Could you check a few things on this model? Use its own coordinates, in mm. A direction names the side the tool comes from. Give positions to 0.01 mm unless a question says otherwise; leave off trailing zeros. Order: outer loops, then holes, each group sorted by start corner. A loop starts at its lowest first (then second) coordinate and runs counter-clockwise, first axis right, second up. Notation, with made-up numbers: M -20.75,54.25 L 17.25,54.25 A9 ccw 17.25,62.25 Z; hole C 67.25,-10.5 d8. An arc over 180 degrees is marked long. Use a Markdown table: item, result. Add a question column.
Item 1: If we mould it in two halves opening along X, with no side actions, what happens to faces 6 (the face through (-6, 6, -22)), 7 (the face through (18.5, 18, 27)), 8 (the face through (11.491, 8, 23))? For each: released by +X, released by -X, zero draft, split by the parting line, or undercut.
Item 2: If I drill on L1, parallel to X at y = 1.25, z = -11; L2, parallel to Z at x = -12, y = 3.25; L3, parallel to X at y = 3, z = 23, over which ranges is the centre line in solid material (lowest first)? Write a range as from..to.
Item 3: Suppose I cut it at B-B on y = 10.25. Write out the boundary of the cut face in (x, z).
Item 4: For faces 1 (the face through (1, 2, 20.9)), 2 (the face through (-6, 11.5, 27)), 3 (the face through (-24, 2, -2)), 4 (the face through (11.5, 2, -2)), 5 (the face through (-7, 16, 24.5)), which set-ups out of +Z, -Z, +X, -X, +Y, -Y let a thin tool reach every point of the face, with its end or its side?
Item 5: Suppose I cut it at D-D on x = -6.5. Write out the boundary of the cut face in (y, z).
Item 6: Suppose I cut it at A-A on y = 6.5. Count the separate pieces of the cut face and the enclosed holes in it, plus the area to 3 significant figures.
Item 7: Suppose I cut it at C-C on z = -13. Write out the boundary of the cut face in (x, y), plus the area to 3 significant figures.
Item 8: I'm going to push flat-ended pins straight in: pin 1 Ø5 at (x, z) = (-36.5, 26) entering from +Y; pin 2 Ø10 at (x, z) = (-2.5, 5) entering from -Y; pin 3 Ø2 at (x, y) = (-4.5, 5) entering from +Z; pin 4 Ø8 at (x, z) = (17, 1.5) entering from +Y. Where does each tip first touch, or does it pass through?
from build123d import *

# Parameters (mm, degrees)
ESQUISSE1_W             = 35.5
ESQUISSE1_H             = 56
ESQUISSE1_W_2           = 20.1
ESQUISSE1_H_2           = 40.9
BOSS_EXTRU_1_DEPTH      = 4
BOSS_EXTRU_2_DEPTH      = 4
BOSS_EXTRU_5_DEPTH      = 4
ESQUISSE10_W            = 17
ESQUISSE10_H            = 13
BOSS_EXTRU_6_DEPTH      = 7
ESQUISSE11_R            = 3
ENL_V_MAT_EXTRU_1_DEPTH = 7
CONG_1_R                = 0.5
ESQUISSE12_W            = 8
ESQUISSE12_H            = 10.6
ENL_V_MAT_EXTRU_2_DEPTH = 11.5


with BuildPart() as part:
    # Esquisse1 → Boss.-Extru.1 (new body)
    with BuildSketch(Plane(origin=(0, 0, 0), x_dir=(1, 0, 0), z_dir=(0, 1, 0))):
        with Locations((-6.25, -0.5)):
            Rectangle(ESQUISSE1_W, ESQUISSE1_H)
        with Locations((-6.05, -0.45)):
            Rectangle(ESQUISSE1_W_2, ESQUISSE1_H_2, mode=Mode.SUBTRACT)
    extrude(amount=BOSS_EXTRU_1_DEPTH)

    # Esquisse5 → Boss.-Extru.2 (add)
    with BuildSketch(Plane.XY.offset(28.5)):
        Polygon((-6.25, 8), (-6.25, 4), (-6.25, 0), (11.5, 0), (11.5, 13), (18.5, 13), (18.5, 18), (18.5, 23), (-6.25, 23), (-6.25, 18), align=None)
    boss_extru_2 = extrude(amount=-BOSS_EXTRU_2_DEPTH)

    # Symétrie1: Boss.-Extru.2 across plane
    add(boss_extru_2.mirror(Plane(origin=(-6.25, 4, 24.5), x_dir=(0, 0, 1), z_dir=(-1, 0, 0))))

    # Esquisse9 → Boss.-Extru.5 (add)
    with BuildSketch(Plane(origin=(0, 4, 0), x_dir=(-1, 0, 0), z_dir=(0, -1, 0))):
        Polygon((18.5, -25.5), (18.5, -23), (18.5, 20), (18.5, 22), (-6, 22), (-6, -25.5), align=None)
    extrude(amount=-BOSS_EXTRU_5_DEPTH)

    # Esquisse10 → Boss.-Extru.6 (add)
    with BuildSketch(Plane.XY.offset(28.5)):
        with Locations((19.990927164, 6.5)):
            Rectangle(ESQUISSE10_W, ESQUISSE10_H)
    boss_extru_6 = extrude(amount=-BOSS_EXTRU_6_DEPTH)

    # Symétrie2: Boss.-Extru.6 across plane
    add(boss_extru_6.mirror(Plane(origin=(-6.25, 0, 0), x_dir=(0, 0, 1), z_dir=(1, 0, 0))))

    # Esquisse11 → Enlèv. mat.-Extru.1 (cut)
    with BuildSketch(Plane(origin=(0, 0, 21.5), x_dir=(-1, 0, 0), z_dir=(0, 0, -1))):
        with Locations((-19.990927164, 6.5)):
            Circle(ESQUISSE11_R)
    enl_v_mat_extru_1 = extrude(amount=-ENL_V_MAT_EXTRU_1_DEPTH, mode=Mode.SUBTRACT)

    # Symétrie3: Enlèv. mat.-Extru.1 across plane
    add(enl_v_mat_extru_1.mirror(Plane(origin=(-6.25, 0, 0), x_dir=(0, 0, 1), z_dir=(1, 0, 0))), mode=Mode.SUBTRACT)

    # Congé1
    cong_1_edges = [part.edges().sort_by_distance(p)[0] for p in [
        (19.995463582, 0, 21.5),
        (11.490927164, 8.5, 24.5),
        (19.990927164, 13, 21.5),
        (28.490927164, 6.5, 21.5),
        (-21.245463582, 4, 24.5),
        (-23.990927164, 8.5, 24.5),
        (-32.495463582, 0, 21.5),
        (-40.990927164, 6.5, 21.5),
        (-32.490927164, 13, 21.5),
        (14.995463582, 13, 24.5),
        (18.5, 13, 26.5),
        (-6.25, 23, 24.5),
        (18.5, 18, 24.5),
        (-31, 13, 26.5),
        (-27.495463582, 13, 24.5),
        (-31, 18, 24.5),
        (8.745463582, 4, 24.5),
        (-6.25, 8, 24.5),
        (6, 6, 24.5),
        (-18.5, 6, 24.5),
    ]]
    fillet(cong_1_edges, radius=CONG_1_R)

    # Esquisse12 → Enlèv. mat.-Extru.2 (cut)
    with BuildSketch(Plane.XZ):
        with Locations((-6.05, 23.2)):
            Rectangle(ESQUISSE12_W, ESQUISSE12_H)
    extrude(amount=-ENL_V_MAT_EXTRU_2_DEPTH, mode=Mode.SUBTRACT)


solid = part.part
Findings below:
| question | item | result |
|---|---|---|
| 1 | face 6 | zero draft |
| 1 | face 7 | released by +X |
| 1 | face 8 | undercut |
| 2 | L1 | x = -24..-16.1, 4..11.5 |
| 2 | L2 | z = -27.5..-20, 20.9..28.5 |
| 2 | L3 | x = -40.99..-10.05, -2.05..28.49 |
| 3 | outline | M -40.99,22 A0.5 ccw -40.49,21.5 L -23.99,21.5 L -23.99,24 A0.5 cw -23.49,24.5 L -10.05,24.5 L -10.05,28.5 L -40.99,28.5 Z; M -2.05,24.5 L 10.99,24.5 A0.5 cw 11.49,24 L 11.49,21.5 L 27.99,21.5 A0.5 ccw 28.49,22 L 28.49,28.5 L -2.05,28.5 Z |
| 4 | face 1 | -Y |
| 4 | face 2 | +Z, -Z, -Y |
| 4 | face 3 | -Z, -X, +Y, -Y |
| 4 | face 4 | -Z, +X, +Y, -Y |
| 4 | face 5 | -Z, +Y |
| 5 | outline | M 0,-27.5 L 4,-27.5 L 4,-22 L 8,-22 L 8,17.9 L 4,17.9 L 4,-20 L 0,-20 Z; M 11.5,24.5 L 22.5,24.5 A0.5 ccw 23,25 L 23,28.5 L 11.5,28.5 Z |
| 6 | separate pieces | 3 |
| 6 | enclosed holes | 0 |
| 6 | area | 1,350 mm^2 |
| 7 | outline | M -24,0 L -16.1,0 L -16.1,4 L 4,4 L 4,0 L 11.5,0 L 11.5,4 L 6,4 L 6,8 L -18.5,8 L -18.5,4 L -24,4 Z |
| 7 | area | 160 mm^2 |
| 8 | pin 1 | stops at y = 13 |
| 8 | pin 2 | stops at y = 4 |
| 8 | pin 3 | stops at z = 17.9 |
| 8 | pin 4 | passes through |
